Design review of the part built by this model. Coordinates are the model's own, in mm. Face numbers are marked on the shaded views. Coordinates: 2 decimals unless noted, no trailing zeros. Write each loop counter-clockwise with the first axis right and the second up, starting at its lowest first coordinate (ties: lowest second). Pieces come first, ordered by that corner, then holes. Notation, with made-up numbers: (-28.75, -23.5) -> (-10.75, -23.5) arc R22 ccw to (-10.75, -3.5) -> close; hole circle Ø8 at (10.25, -38.75). An arc over 180 degrees is marked (long way). One line per question, with ' | ' between items. Start each with the question number.
Q1. Draft analysis for pull direction Z (two halves, no side actions). For the marked faces 1, 2, 3 and 4, state which applies: pulls with the +Z half, pulls with the -Z half, needs draft (parallel to the pull), parting line crosses it, or undercut.
Q2. For P1, Ø2, axis at y = -18.4, z = 7.75, coming from the -X side, flat-tipped, find the tip position at first contact; note if it passes through.
Q3. Add section A-A on x = -24. State the section outline as (y, z) points, and give its area (3 significant figures).
Q4. Wall thickness on probe 1 along X at (y, z) = (14, 14.25); probe 2 along X at (y, z) = (21, 15); probe 3 along Y at (x, z) = (-24.5, 7.5): over which ranges is each line inside the solid? List them lowest first.
Q5. Add section B-B on z = 4.5. State the section outline as (x, y) points.
from build123d import *

# Parameters (mm, degrees)
SALIENTE_EXTRUIR1_DEPTH = 18
CORTAR_EXTRUIR1_DEPTH   = 0.5
CROQUIS3_R              = 1.25
CROQUIS3_W              = 12
CROQUIS3_H              = 15
CORTAR_EXTRUIR2_DEPTH   = 0.5


with BuildPart() as part:
    # Croquis1 → Saliente-Extruir1 (new body)
    with BuildSketch(Plane.XY):
        with BuildLine():
            Line((20.5, -28.5), (-22.5, -28.5))
            ThreePointArc((-22.5, -28.5), (-26.742640687, -26.742640687), (-28.5, -22.5))
            Line((-28.5, -22.5), (-28.5, 20.5))
            ThreePointArc((-28.5, 20.5), (-26.156854249, 26.156854249), (-20.5, 28.5))
            Line((-20.5, 28.5), (20.5, 28.5))
            ThreePointArc((20.5, 28.5), (26.156854249, 26.156854249), (28.5, 20.5))
            Line((28.5, 20.5), (28.5, -20.5))
            ThreePointArc((28.5, -20.5), (26.156854249, -26.156854249), (20.5, -28.5))
        make_face()
    extrude(amount=SALIENTE_EXTRUIR1_DEPTH)

    # Croquis2 → Cortar-Extruir1 (cut)
    with BuildSketch(Plane.XY.offset(18)):
        with BuildLine():
            Line((20.5, 26.5), (-20.5, 26.5))
            ThreePointArc((-20.5, 26.5), (-24.742640687, 24.742640687), (-26.5, 20.5))
            Line((-26.5, 20.5), (-26.5, -22.5))
            ThreePointArc((-26.5, -22.5), (-25.328427125, -25.328427125), (-22.5, -26.5))
            Line((-22.5, -26.5), (20.5, -26.5))
            ThreePointArc((20.5, -26.5), (24.742640687, -24.742640687), (26.5, -20.5))
            Line((26.5, -20.5), (26.5, 20.5))
            ThreePointArc((26.5, 20.5), (24.742640687, 24.742640687), (20.5, 26.5))
        make_face()
        with BuildLine():
            Line((-26, 20.5), (-26, -22.5))
            ThreePointArc((-26, -22.5), (-24.974873734, -24.974873734), (-22.5, -26))
            Line((-22.5, -26), (20.5, -26))
            ThreePointArc((20.5, -26), (24.389087297, -24.389087297), (26, -20.5))
            Line((26, -20.5), (26, 20.5))
            ThreePointArc((26, 20.5), (24.389087297, 24.389087297), (20.5, 26))
            Line((20.5, 26), (-20.5, 26))
            ThreePointArc((-20.5, 26), (-24.389087297, 24.389087297), (-26, 20.5))
        make_face(mode=Mode.SUBTRACT)
    extrude(amount=-CORTAR_EXTRUIR1_DEPTH, mode=Mode.SUBTRACT)

    # Croquis3 → Cortar-Extruir2 (cut)
    with BuildSketch(Plane.ZY.offset(28.5)):
        with Locations((7.75, -18.4)):
            Circle(CROQUIS3_R)
        with Locations((9, 9)):
            Rectangle(CROQUIS3_W, CROQUIS3_H)
        Polygon((9, -3.5), (7.3, -3.5), (5.7, -5.1), (5.7, -10.3), (7.3, -11.9), (9, -11.9), align=None)
    extrude(amount=-CORTAR_EXTRUIR2_DEPTH, mode=Mode.SUBTRACT)


solid = part.part
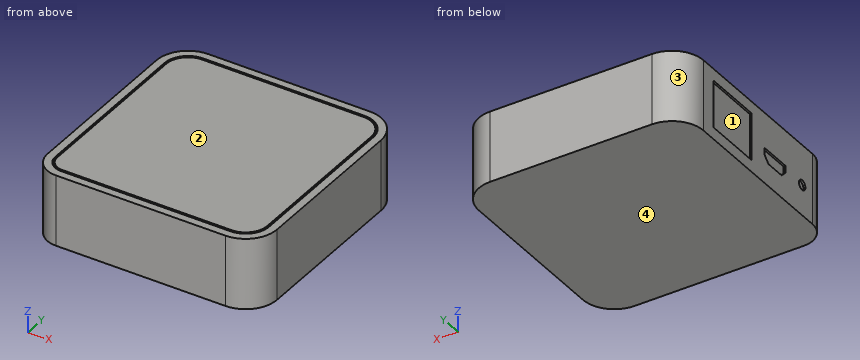
Output values:
1) face 1: undercut | face 2: pulls with the +Z half | face 3: needs draft | face 4: pulls with the -Z half
2) P1: stops at x = -28
3) outline: (-28.31, 0) -> (27.69, 0) -> (27.69, 18) -> (25.37, 18) -> (25.37, 17.5) -> (24.74, 17.5) -> (24.74, 18) -> (-25.66, 18) -> (-25.66, 17.5) -> (-26.21, 17.5) -> (-26.21, 18) -> (-28.31, 18) -> close | area: 1,010 mm2
4) probe 1: x = -28 to 28.5 | probe 2: x = -28.48 to 28.48 | probe 3: y = -28.16 to 27.43
5) outline: (-28.5, -22.5) arc R6 ccw to (-22.5, -28.5) -> (20.5, -28.5) arc R8 ccw to (28.5, -20.5) -> (28.5, 20.5) arc R8 ccw to (20.5, 28.5) -> (-20.5, 28.5) arc R8 ccw to (-28.5, 20.5) -> (-28.5, 16.5) -> (-28, 16.5) -> (-28, 1.5) -> (-28.5, 1.5) -> close
